Check sheet for the modelled part. Datum: model origin and axes. Units: mm. Face numbers are marked on the shaded views. A direction names the side the tool comes from. Round coordinates to 2 decimals unless told otherwise and drop trailing zeros. Write each loop counter-clockwise with the first axis right and the second up, starting at its lowest first coordinate (ties: lowest second). Pieces come first, ordered by that corner, then holes. Notation, with made-up numbers: (-18.5, -4.75) - (12.5, -4.75) arc R34 ccw to (12.5, 26.25) - close; hole circle Ø6 at (87.5, 51.5). An arc over 180 degrees is marked (long way). Use one line per item in the form item = value. Start each with the question number.
1) Section check A-A (y = 0.2). Record the boundary of the cut face in (x, z), then the cut area to 3 significant figures.
2) Section check C-C (x = -14). Record the boundary of the cut face in (y, z), then the cut area to 3 significant figures.
3) Scan lines: probe 1 along Z at (x, y) = (14, 0.65); probe 2 along X at (y, z) = (0.55, 2.5); probe 3 along X at (y, z) = (0.5, 2.75). Record each from-to range of solid material in increasing order.
4) Section check D-D (z = -1). Record the boundary of the cut face in (x, y).
5) Gauge pin test, flat end, axial feed: P1, Ø4, axis at x = 4, z = -1.5, coming from the +Y side. Record the tip position at first contact, or that the pin passes through.
6) Section check B-B (z = -2.5). Record the boundary of the cut face in (x, y).
7) Set-up check for the marked faces 1 and 2: record each of +Z, -Z, +X, -X, +Y, -Y from which the full face is reachable in a straight line by a thin tool's end or side.
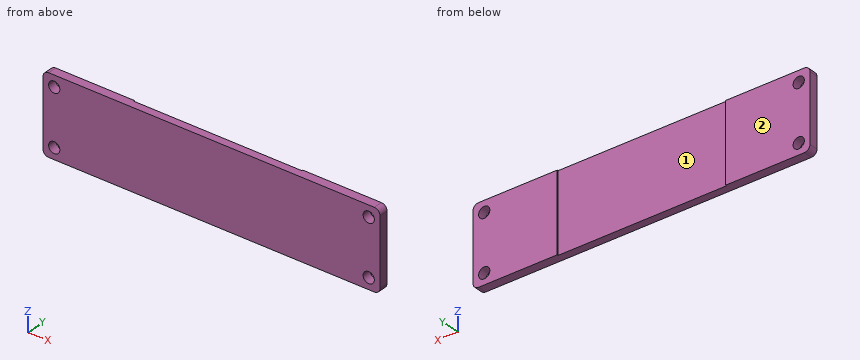
from build123d import *

# Parameters (mm, degrees)
SKETCH_1_W          = 30
SKETCH_1_H          = 7
EXTRUDE_1_DEPTH     = 0.8
SKETCH_2_R          = 0.5
CUT_EXTRUDE_1_DEPTH = 1.8
FILLET_1_R          = 0.5
SKETCH_3_W          = 15
SKETCH_3_H          = 7
CUT_EXTRUDE_2_DEPTH = 0.1


with BuildPart() as part:
    # 草图1 → 凸台-拉伸1 (new body)
    with BuildSketch(Plane(origin=(0, 0, 0), x_dir=(1, 0, 0), z_dir=(0, 1, 0))):
        Rectangle(SKETCH_1_W, SKETCH_1_H)
    extrude(amount=EXTRUDE_1_DEPTH)

    # 草图2 → 切除-拉伸1 (cut, through all)
    with BuildSketch(Plane(origin=(0, 0.8, 0), x_dir=(1, 0, 0), z_dir=(0, 1, 0))):
        with Locations((-14, 2.5)):
            Circle(SKETCH_2_R)
        with Locations((14, 2.5)):
            Circle(SKETCH_2_R)
        with Locations((14, -2.5)):
            Circle(SKETCH_2_R)
        with Locations((-14, -2.5)):
            Circle(SKETCH_2_R)
    extrude(amount=-CUT_EXTRUDE_1_DEPTH, mode=Mode.SUBTRACT)

    # 圆角1
    fillet_1_edges = [part.edges().sort_by_distance(p)[0] for p in [
        (-15, 0.4, -3.5),
        (15, 0.4, -3.5),
        (15, 0.4, 3.5),
        (-15, 0.4, 3.5),
    ]]
    fillet(fillet_1_edges, radius=FILLET_1_R)

    # 草图3 → 切除-拉伸2 (cut)
    with BuildSketch(Plane(origin=(0, 0.8, 0), x_dir=(1, 0, 0), z_dir=(0, 1, 0))):
        Rectangle(SKETCH_3_W, SKETCH_3_H)
    extrude(amount=-CUT_EXTRUDE_2_DEPTH, mode=Mode.SUBTRACT)


solid = part.part
Results are:
q1.outline = (-15, -3) arc R0.5 ccw to (-14.5, -3.5) - (14.5, -3.5) arc R0.5 ccw to (15, -3) - (15, 3) arc R0.5 ccw to (14.5, 3.5) - (-14.5, 3.5) arc R0.5 ccw to (-15, 3) - close; hole circle Ø1 at (-14, -2.5); hole circle Ø1 at (-14, 2.5); hole circle Ø1 at (14, -2.5); hole circle Ø1 at (14, 2.5)
q1.area = 207 mm²
q2.outline = (0, -3.5) - (0.8, -3.5) - (0.8, -3) - (0, -3) - close; (0, -2) - (0.8, -2) - (0.8, 2) - (0, 2) - close; (0, 3) - (0.8, 3) - (0.8, 3.5) - (0, 3.5) - close
q2.area = 4.00 mm²
q3.probe_1 = -3.5 to -3, -2 to 2, 3 to 3.5
q3.probe_2 = -15 to -14.5, -13.5 to 13.5, 14.5 to 15
q3.probe_3 = -15 to -14.43, -13.57 to 13.57, 14.43 to 15
q4.outline = (-15, 0) - (15, 0) - (15, 0.8) - (7.5, 0.8) - (7.5, 0.7) - (-7.5, 0.7) - (-7.5, 0.8) - (-15, 0.8) - close
q5.P1 = 0.7
q6.outline = (-15, 0) - (-14.5, 0) - (-14.5, 0.8) - (-15, 0.8) - close; (-13.5, 0) - (13.5, 0) - (13.5, 0.8) - (7.5, 0.8) - (7.5, 0.7) - (-7.5, 0.7) - (-7.5, 0.8) - (-13.5, 0.8) - close; (14.5, 0) - (15, 0) - (15, 0.8) - (14.5, 0.8) - close
q7.face_1 = +Z, -Z, +Y
q7.face_2 = +Z, -Z, +X, -X, +Y
